Solid Edge part; units mm, degrees
sketch "Sketch1" plane through (0, 0, 0) normal (0, 0, 1) x (1, 0, 0)
  line L0 (-13.5647, 21) -> (-13.5647, -21)
  line L1 (20, 15) -> (20, -15)
  arc A0 (-13.5647, 21) -> (20, 15) centre (0, 0) cw
  arc A1 (-13.5647, -21) -> (20, -15) centre (0, 0) ccw
  dimension "D1" = 13.5647
  dimension "D2" = 20
extrude "Protrusion1" add sketch "Sketch1" along normal blind 40
shell "Espesor_1" thickness 1.5 removed faces 1 at (-8.3062, -16.1667, 40)
hole "Agujero_1" at (-13.5647, 13, 30) direction (1, 0, 0) diameter 16 end up to next
hole "Hole1" at (-13.5647, -13, 30) direction (1, 0, 0) diameter 16 end up to next
sketch "Sketch2" plane through (-13.5647, 0, 20) normal (-1, 0, 0) x (0, -1, 0)
  line L0 (0, 3.3123) -> (-7.8596, -5.4456)
  line L1 (-7.8596, -5.4456) -> (4.9404, -5.4456)
  line L2 (4.9404, -5.4456) -> (4.9404, -3.6491)
  line L3 (4.9404, -3.6491) -> (-3.9298, -3.6491)
  line L4 (-3.9298, -3.6491) -> (1.2214, 2.0908)
  line L5 (1.2214, 2.0908) -> (0, 3.3123)
  line L6 (9.75, -13.7333) -> (12.75, -13.7333)
  line L7 (12.75, -13.7333) -> (12.75, -11.7333)
  line L8 (12.75, -11.7333) -> (9.75, -11.7333)
  line L9 (9.75, -11.7333) -> (9.75, -13.7333)
  line L10 (-12.75, -11.7333) -> (-12.75, -13.7333)
  line L11 (-12.75, -13.7333) -> (-9.75, -13.7333)
  line L12 (-9.75, -11.7333) -> (-9.75, -13.7333)
  line L13 (-9.75, -11.7333) -> (-12.75, -11.7333)
  line L14 (-8.25, -13.7333) -> (-8.25, -11.7333)
  line L15 (-5.25, -11.7333) -> (-8.25, -11.7333)
  line L16 (-5.25, -11.7333) -> (-5.25, -13.7333)
  line L17 (-8.25, -13.7333) -> (-5.25, -13.7333)
  line L18 (-0.75, -11.7333) -> (-0.75, -13.7333)
  line L19 (-3.75, -13.7333) -> (-0.75, -13.7333)
  line L20 (-3.75, -11.7333) -> (-3.75, -13.7333)
  line L21 (-0.75, -11.7333) -> (-3.75, -11.7333)
  line L22 (8.25, -13.7333) -> (8.25, -11.7333)
  line L23 (8.25, -11.7333) -> (5.25, -11.7333)
  line L24 (5.25, -11.7333) -> (5.25, -13.7333)
  line L25 (5.25, -13.7333) -> (8.25, -13.7333)
  line L26 (0.75, -11.7333) -> (0.75, -13.7333)
  line L27 (0.75, -13.7333) -> (3.75, -13.7333)
  line L28 (3.75, -11.7333) -> (3.75, -13.7333)
  line L29 (3.75, -11.7333) -> (0.75, -11.7333)
extrude "Cutout1" cut sketch "Sketch2" against normal up to next
sketch "Sketch3" plane through (3.2177, 0, 1.5) normal (0, 0, 1) x (0, -1, 0)
  line L0 (15, 13.7823) -> (-15, 13.7823)
  line L1 (-15, 13.7823) -> (-15, 16.7823)
  line L2 (-15, 16.7823) -> (15, 16.7823)
  line L3 (15, 16.7823) -> (15, 13.7823)
extrude "Cutout2" cut sketch "Sketch3" along normal up to next
For this review, take the finished solid that the model builds, in its own axes (mm). A direction names the side the tool comes from. Round coordinates to 2 decimals unless told otherwise and drop trailing zeros. Write each loop counter-clockwise with the first axis right and the second up, starting at its lowest first coordinate (ties: lowest second). Pieces come first, ordered by that corner, then holes. Notation, with made-up numbers: (53.25, -36) -> (57.25, -36) arc R12 ccw to (57.25, -20) -> close; hole circle Ø1 at (-34.75, 12). An arc over 180 degrees is marked (long way). One line per question, with ' | ' between items. Start each with the question number.
1) For pin 1 Ø6 at (x, z) = (-8, 35) entering from +Y; pin 2 Ø3 at (x, z) = (-5.5, 22) entering from -Y; pin 3 Ø12 at (y, z) = (9.5, 26.5) entering from +X, all flat-tipped, find the tip position at first contact; note any pin that passes through.
2) Add section A-A (y = -2). Write out the cut boundary in (x, z), and give its area (3 significant figures).
3) Add section B-B (z = 5). Write out the cut boundary in (x, y), and give its area (3 significant figures).
4) Wall thickness on line 1 along Z through (x, y) = (-12.6, 13); line 2 along Y through (x, z) = (0, 14); line 3 along X through (y, z) = (6.5, 3.5): over which ranges is each line inside the solid? List them lowest first.
5) Add section C-C (y = 19.5). Write out the cut boundary in (x, z).
6) Add section D-D (z = 24). Write out the cut boundary in (x, y), and give its area (3 significant figures).
7) Mouldability with a two-part tool opening along Y and no side actions: class faces 5 (the flat face through (-13.565, 0, 20)), 6 (the flat face through (-12.83, -0.62, 22.69)) as +Y half, -Y half, draft (parallel to the pull), parting line (faces both ways), or undercut.
8) Machinability: for faces 1 (the flat face through (-13, 0, 40)), 2 (the flat face through (19, 15, 20)), 3 (the flat face through (-12.065, 5, 20)), 4 (the flat face through (-13, 11, 8.267)), which of the approach directions +Z, -Z, +X, -X, +Y, -Y give a long, thin tool a straight path to every point of the face, cutting with its end or side? Answer none if there is none.
Reported:
1) pin 1: stops at y = 24.49 | pin 2: stops at y = -24.68 | pin 3: stops at x = 20
2) outline: (-13.56, 0) -> (20, 0) -> (20, 1.5) -> (-12.06, 1.5) -> (-12.06, 6.27) -> (-13.56, 6.27) -> close; (-13.56, 8.27) -> (-12.06, 8.27) -> (-12.06, 14.55) -> (-13.56, 14.55) -> close; (-13.56, 16.35) -> (-12.06, 16.35) -> (-12.06, 40) -> (-13.56, 40) -> close | area: 102 mm²
3) outline: (-13.56, -21) arc R25 ccw to (20, -15) -> (18.09, -15) arc R23.5 cw to (-12.06, -20.17) -> (-12.06, 20.17) arc R23.5 cw to (18.09, 15) -> (20, 15) arc R25 ccw to (-13.56, 21) -> close | area: 168 mm²
4) line 1: z = 0 to 22, 38 to 40 | line 2: y = -25 to -23.5, 23.5 to 25 | line 3: x = -13.56 to -12.06
5) outline: (-13.56, 0) -> (15.64, 0) -> (15.64, 40) -> (13.11, 40) -> (13.11, 1.5) -> (-12.06, 1.5) -> (-12.06, 25.34) -> (-13.56, 25.34) -> close; (-13.56, 34.66) -> (-12.06, 34.66) -> (-12.06, 40) -> (-13.56, 40) -> close
6) outline: (-13.56, -21) arc R25 ccw to (20, -15) -> (18.09, -15) arc R23.5 cw to (-12.06, -20.17) -> (-12.06, -18.29) -> (-13.56, -18.29) -> close; (-13.56, -7.71) -> (-12.06, -7.71) -> (-12.06, 7.71) -> (-13.56, 7.71) -> close; (-13.56, 18.29) -> (-12.06, 18.29) -> (-12.06, 20.17) arc R23.5 cw to (18.09, 15) -> (20, 15) arc R25 ccw to (-13.56, 21) -> close | area: 136 mm²
7) face 5: draft | face 6: undercut
8) face 1: +Z, +X, -X, +Y, -Y | face 2: +Z, +X | face 3: +Z | face 4: +X, -X
